Autodesk Inventor part; units mm, degrees
ref_plane "YZ Plane" through (0, 0, 0) normal (1, 0, 0) x (0, 1, 0)
ref_plane "XZ Plane" through (0, 0, 0) normal (0, 1, 0) x (-1, 0, 0)
ref_plane "XY Plane" through (0, 0, 0) normal (0, 0, 1) x (1, 0, 0)
sketch "Sketch1" plane through (0, 0, 0) normal (0, 0, 1) x (1, 0, 0)
  circle A0 centre (0, 6.647) radius 1.75
  point P0 (0, 0)
  dimension "d0" = 3.5
  dimension "d1" = 6.647
extrude "Extrusion1" add sketch "Sketch1" against normal blind 2
pattern_circular "Circular Pattern1" count 3 over 360 about axis through (0, 0, -10) along (0, 0, 1) of "Extrusion1"
sketch "Sketch3" plane through (-5.7565, -3.3235, 0) normal (0, 0, 1) x (1, 0, 0)
  circle A0 centre (5.7565, 3.3235) radius 10.3482
  circle A1 centre (5.7565, 3.3235) radius 11.0482
  dimension "d13" = 0.7
extrude "Extrusion3" add sketch "Sketch3" along normal blind 2 contours A0
properties part number "PSteg"
Work out the finished part from the listing and answer in its coordinate system (mm). A direction names the side the tool comes from. Round coordinates to 2 decimals unless told otherwise and drop trailing zeros. Order: outer loops, then holes, each group sorted by start corner. A loop starts at its lowest first (then second) coordinate and runs counter-clockwise, first axis right, second up.
Q1. A tool of negligible diameter and unlimited length cuts with its end or side. For faces 5 (the cylindrical face through (9.87, -3.11, 0.99)), 6 (the flat face through (0, 0, 0)), from which of +Z, -Z, +X, -X, +Y, -Y can it reach the whole face along a straight path? Write none if from no direction.
Solution:
face 5: +Z, -Z
face 6: -Z
Q2. A cutting plane is placed at D-D, the plane z = 0.8. Determine the outline of the cut face in (x, y), then the cut area to 3 significant figures.
Solution:
outline: circle Ø20.7 at (0, 0)
area: 336 mm2
Q3. The mould has two halves that part along X. Classify faces 1 (the flat face through (-6, -3, -2)), 2 (the cylindrical face through (7.426, -2.798, -0.986)), 3 (the cylindrical face through (-4.14, -3.99, -0.99)), 4 (the cylindrical face through (-0.38, 4.94, -0.99)): pulls with the +X half, pulls with the -X half, needs draft (parallel to the pull), parting line crosses it, or undercut.
Solution:
face 1: needs draft
face 2: undercut
face 3: undercut
face 4: parting line crosses it
Q4. A cutting plane is placed at A-A, the plane x = 0. Determine the outline of the cut face in (y, z).
Solution:
outline: (-10.35, 0) - (4.9, 0) - (4.9, -2) - (8.4, -2) - (8.4, 0) - (10.35, 0) - (10.35, 2) - (-10.35, 2) - close
Q5. A cutting plane is placed at C-C, the plane z = -0.6. Determine the outline of the cut face in (x, y), then the cut area to 3 significant figures.
Solution:
outline: circle Ø3.5 at (-5.76, -3.32); circle Ø3.5 at (0, 6.65); circle Ø3.5 at (5.76, -3.32)
area: 28.9 mm2
Q6. Find the intervals of material crossed by line 1 along Z through (x, y) = (-6.5, 8); line 2 along X through (y, z) = (-4, -1.6); line 3 along X through (y, z) = (7, 1.05), in increasing order.
Solution:
line 1: z = 0 to 2
line 2: x = -7.37 to -4.14, 4.14 to 7.37
line 3: x = -7.62 to 7.62
Q7. A cutting plane is placed at B-B, the plane y = 5.75. Determine the outline of the cut face in (x, z), then the cut area to 3 significant figures.
Solution:
outline: (-8.6, 0) - (-1.5, 0) - (-1.5, -2) - (1.5, -2) - (1.5, 0) - (8.6, 0) - (8.6, 2) - (-8.6, 2) - close
area: 40.4 mm2
Q8. Given pin 1 Ø3 at (x, y) = (-3, -4) entering from -Z; pin 2 Ø1.5 at (y, z) = (6.5, -1) entering from -X, each flat-ended and moving along its own axis, determine where each tip first touches the part or whether it passes through.
Solution:
pin 1: stops at z = -2
pin 2: stops at x = -1.75
